Here's how the part is built. I have some questions about the finished solid (model axes, mm). Face numbers are marked on the shaded views. A direction names the side the tool comes from. Round coordinates to 2 decimals unless told otherwise and drop trailing zeros. Write each loop counter-clockwise with the first axis right and the second up, starting at its lowest first coordinate (ties: lowest second). Pieces come first, ordered by that corner, then holes. Notation, with made-up numbers: (39, 80) - (92, 80) arc R19 ccw to (92, 92) - close; hole circle Ø6 at (12, 0.5). An arc over 180 degrees is marked (long way). Use one line per item in the form item = value. Start each with the question number.
1. Will these pins go through, and if not, where does the flat tip stop? pin 1 (0.9 mm diameter, centred on y = 33.5, z = 2, fed in from -X); pin 2 (0.9 mm diameter, centred on x = -1.5, z = 2, fed in from +Y); pin 3 (1.2 mm diameter, centred on x = -5, z = 1, fed in from +Y).
2. I want a section at B-B, the plane z = 1.4. State how many separate pieces and enclosed holes the cut face has, plus the area to 3 significant figures.
3. I want a section at D-D, the plane y = 12.5. List the corners of the cut face in (x, z) for me, plus the area to 3 significant figures.
4. We'd pull the mould along Y, two halves only. Please class the marked faces 1, 2 and 3: +Y half, -Y half, draft (parallel to the pull), parting line (faces both ways), or undercut.
5. Which directions (+Z, -Z, +X, -X, +Y, -Y) give clear straight access to the entire face, cutting with the end or side of a thin tool? Please do the marked faces 4 and 5.
6. If I drill on line 1 along Y through (x, z) = (0, 1.3); line 2 along Y through (x, z) = (-4.75, 0.45); line 3 along X through (y, z) = (33.5, 1.75), over which ranges is the centre line in solid material (lowest first)?
7. I want a section at C-C, the plane x = -7.5. List the corners of the cut face in (y, z) for me, plus the area to 3 significant figures.
8. I want a section at A-A, the plane y = 4. List the corners of the cut face in (x, z) for me, plus the area to 3 significant figures.
```python
from build123d import *

# Parameters (mm, degrees)
CROQUIS2_R              = 1.5
CROQUIS2_R_2            = 1
SALIENTE_EXTRUIR1_DEPTH = 3


with BuildPart() as part:
    # Croquis2 → Saliente-Extruir1 (new body)
    with BuildSketch(Plane.XY):
        with BuildLine():
            Line((10, 0), (10, 30))
            add(Edge.make_bspline(
                [(10, 40), (13.382456464, 40), (10, 31.604422757), (10, 30)],
                knots=[0, 0, 0, 0, 1, 1, 1, 1], degree=3))
            ThreePointArc((10, 40), (7.878679656, 40.878679656), (7, 43))
            Line((7, 43), (7, 50))
            Line((7, 50), (5, 50))
            Line((5, 50), (5, 45))
            ThreePointArc((5, 45), (3.535533906, 41.464466094), (0, 40))
            ThreePointArc((0, 40), (-1.767766953, 39.267766953), (-2.5, 37.5))
            Line((-2.5, 37.5), (-2.5, 37.4))
            ThreePointArc((-2.5, 37.4), (-3.202943725, 35.702943725), (-4.9, 35))
            Line((-4.9, 35), (-6, 35))
            Line((-6, 35), (-6, 30))
            Line((-6, 30), (6, 30))
            Line((6, 30), (6, 7))
            Line((6, 7), (-10, 7))
            Line((-10, 7), (-10, 0))
            Line((-10, 0), (-10, -6))
            Line((-10, -6), (10, -6))
            Line((10, -6), (10, 0))
        make_face()
        with Locations((0, 37.5)):
            Circle(CROQUIS2_R, mode=Mode.SUBTRACT)
        with Locations((0, 33)):
            Circle(CROQUIS2_R_2, mode=Mode.SUBTRACT)
        with Locations((0, 4)):
            Circle(CROQUIS2_R_2, mode=Mode.SUBTRACT)
    extrude(amount=SALIENTE_EXTRUIR1_DEPTH)


solid = part.part
```
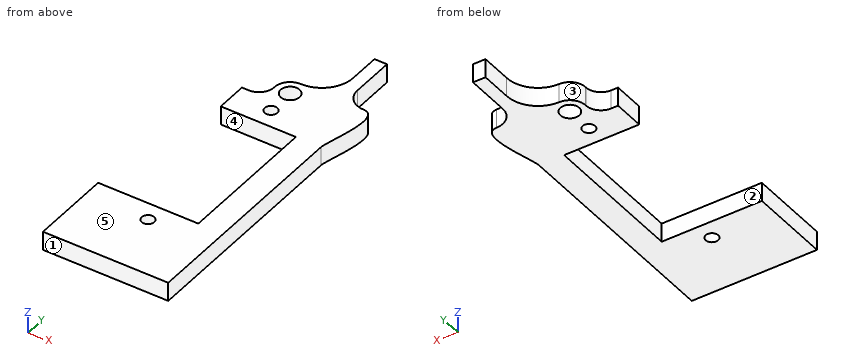
Model answer:
q1.pin_1 = -6
q1.pin_2 = 39.77
q1.pin_3 = 35.05
q2.separate_pieces = 1
q2.enclosed_holes = 3
q2.area = 518 mm2
q3.outline = (6, 0) - (10, 0) - (10, 3) - (6, 3) - close
q3.area = 12.0 mm2
q4.face_1 = -Y half
q4.face_2 = undercut
q4.face_3 = +Y half
q5.face_4 = +Z, -Z, -X
q5.face_5 = +Z, +X, -X, +Y, -Y
q6.line_1 = -6 to 3, 5 to 7, 30 to 32, 34 to 36, 39 to 40
q6.line_2 = -6 to 7, 30 to 35
q6.line_3 = -6 to -0.87, 0.87 to 10.8
q7.outline = (-6, 0) - (7, 0) - (7, 3) - (-6, 3) - close
q7.area = 39.0 mm2
q8.outline = (-10, 0) - (-1, 0) - (-1, 3) - (-10, 3) - close; (1, 0) - (10, 0) - (10, 3) - (1, 3) - close
q8.area = 54.0 mm2
